Read the model definition and answer for the solid it produces. Units are mm, in the model's axes. A direction names the side the tool comes from. Coordinates: 2 decimals unless noted, no trailing zeros. Write each loop counter-clockwise with the first axis right and the second up, starting at its lowest first coordinate (ties: lowest second). Pieces come first, ordered by that corner, then holes.
Autodesk Inventor part; units mm, degrees
ref_plane "YZ Plane" through (0, 0, 0) normal (1, 0, 0) x (0, 1, 0)
ref_plane "XZ Plane" through (0, 0, 0) normal (0, 1, 0) x (-1, 0, 0)
ref_plane "XY Plane" through (0, 0, 0) normal (0, 0, 1) x (1, 0, 0)
sketch "Sketch1" plane through (0, 0, 0) normal (1, 0, 0) x (0, 1, 0)
  circle A0 centre (0, 0) radius 3.85
  dimension "d0" = 7.7
extrude "Extrusion1" add sketch "Sketch1" along normal blind 5
sketch "Sketch2" plane through (5, 0, 0) normal (1, 0, 0) x (0, 0, -1)
  circle A0 centre (0, 0) radius 3.85
  dimension "d3" = 7.7
extrude "Extrusion2" add sketch "Sketch2" along normal blind 28.5
sketch "Sketch5" plane through (0, 0, 0) normal (-1, 0, 0) x (0, 0, 1)
  circle A0 centre (0, 0) radius 2.4
  line L0 (0, 0) -> (-2.4, 0)
  line L1 (-2.4, 0) -> (-2.4, 2.4)
  line L2 (-2.4, 2.4) -> (0, 2.4)
  line L3 (0, 2.4) -> (0, 0)
  line L4 (-2.4, 2.4) -> (2.4, 2.4)
  line L5 (2.4, 2.4) -> (2.4, -2.4)
  line L6 (2.4, -2.4) -> (-2.4, -2.4)
  line L7 (-2.4, -2.4) -> (-2.4, 2.4)
  line L8 (-2.4, 2.4) -> (2.4, 0)
  line L9 (-2.4, -2.4) -> (2.4, 0)
  line L10 (-2.4, 0) -> (2.4, 2.4)
  line L11 (-2.4, 0) -> (2.4, -2.4)
  line L12 (0, 2.4) -> (2.4, -2.4)
  line L13 (-2.4, -2.4) -> (0, 2.4)
  line L14 (-2.4, 2.4) -> (0, -2.4)
  line L15 (0, -2.4) -> (2.4, 2.4)
  point P0 (1.44, -0.48)
  point P1 (1.44, 0.48)
  point P2 (0.48, 1.44)
  point P3 (-0.48, 1.44)
  point P4 (-1.44, 0.48)
  point P5 (-1.44, -0.48)
  point P6 (-0.48, -1.44)
  point P7 (0.48, -1.44)
  dimension "d23" = 4.8
extrude "Extrusion5" cut sketch "Sketch5" against normal blind 10 contours L9 L12 L15 L8 | L15 L8 L12 L10 A0 | A0 L10 L15 | L12 L11 A0 | A0 L11 L15 L9 L12 | L15 L12 L8 | L9 L15 L12 | L12 L10 L3 | L3 L8 L13 | L14 L9 L11 L15 | L12 L15 L9 L11 L14 L0 L3 L8 | L8 L10 L12 | L15 L11 L9 | L8 L13 L10 L14 A0 | A0 L14 L8 | L10 L13 L8 | L3 L0 L13 L10 | L9 L13 A0 | A0 L13 L11 L14 L9 | L14 L11 L9 | L10 L14 L0 | L0 L13 L11 | L13 L14 L10 | L11 L13 L14
sketch "Sketch7" plane through (0, 0, 0) normal (-1, 0, 0) x (0, 0, 1)
  circle A0 centre (0, 0) radius 3.85
extrude "Extrusion7" cut sketch "Sketch7" against normal blind 2
mirror "Mirror1" about plane through (33.5, 0, 0) normal (1, 0, 0)
properties part number "gear_shaft"
Item 1: The part is cut by section A-A (x = 23.5). Give the vertices of the cut face in (y, z), and give its area (3 significant figures).
Item 2: Find the intervals of material crossed by probe 1 along Y at (x, z) = (60, 3); probe 2 along X at (y, z) = (-1.5, -1.75), in increasing order.
Item 3: For faces 3 (the flat face through (57, 0, 0)), 4 (the flat face through (65, -1, -2)), determine the directions among +Z, -Z, +X, -X, +Y, -Y from which every point of the face is accessible in a straight line to the end or side of a thin tool.
Item 4: Determine the mould class of faces 1 (the flat face through (61.1, -1.4, -1.9)), 2 (the flat face through (2, -1, 2)) for opening direction Z: +Z half, -Z half, draft (parallel to the pull), parting line (faces both ways), or undercut.
Item 5: Given pin 1 (4 mm diameter, centred on x = 9.5, z = 2.5, fed in from -Y), flat-ended and moving along its own axis, determine where the tip first touches the part or whether it passes through.
Answer:
1. outline: circle Ø7.7 at (0, 0)
1. area: 46.6 mm2
2. probe 1: y = -2.41 to 2.41
2. probe 2: x = 10 to 57
3. face 3: +X
3. face 4: +Z, -Z, +X, +Y, -Y
4. face 1: undercut
4. face 2: draft
5. pin 1: stops at y = -3.82
